from build123d import *

# Parameters (mm, degrees)
F0_R     = 4
F0_R_2   = 1.5
F1_DEPTH = 2
F2_DEPTH = 15
F3_SIZE  = 0.5
F4_W     = 2
F4_H     = 1
F5_DEPTH = 4.001
F6_DEPTH = 25.4


with BuildPart() as f1:
    # F0 (on Top) → F1 (new body)
    with BuildSketch(Plane.XY):
        Circle(F0_R)
        Circle(F0_R_2, mode=Mode.SUBTRACT)
    extrude(amount=F1_DEPTH)

    # F0 (on Top) → F2 (join)
    with BuildSketch(Plane.XY):
        Circle(F0_R_2)
    extrude(amount=F2_DEPTH)

    # F3
    f3_edges = [f1.edges().sort_by_distance(p)[0] for p in [
        (-4, 0, 2),
    ]]
    chamfer(f3_edges, length=F3_SIZE)

    # F4 (on Front) → F5 (cut, through all)
    with BuildSketch(Plane.XZ):
        with Locations((0.083052, 13.76275)):
            Rectangle(F4_W, F4_H)
    extrude(amount=-F5_DEPTH, mode=Mode.SUBTRACT)

    # F4 (on Front) → F6 (cut)
    with BuildSketch(Plane.XZ):
        with Locations((0.083052, 13.76275)):
            Rectangle(F4_W, F4_H)
    extrude(amount=F6_DEPTH, mode=Mode.SUBTRACT)


solid = f1.part
Input: part model. Units: mm. Frame: model coordinates. A direction names the side the tool comes from. Coordinates: 2 decimals unless noted, no trailing zeros. Order: outer loops, then holes, each group sorted by start corner. A loop starts at its lowest first (then second) coordinate and runs counter-clockwise, first axis right, second up. Notation, with made-up numbers: M 69.25,68 L 127.25,68 A18 ccw 127.25,88 Z; hole C 29.5,84 d3. An arc over 180 degrees is marked long. One line per question, with ' | ' between items.
Item 1: Pin query (flat end, axial travel): pin 1 (0.8 mm diameter, centred on y = 0, z = 13.5, fed in from +X); pin 2 (3 mm diameter, centred on x = -2.5, z = 9.5, fed in from +Y); pin 3 (4 mm diameter, centred on x = 0, z = 8.5, fed in from +Y). Return the tip coordinate at first contact, or that it passes through.
Geometry results:
pin 1: stops at x = 1.5 | pin 2: stops at y = 1.12 | pin 3: stops at y = 1.5
Item 2: Ray query, line 1 along Z through (x, y) = (-0.5, 0.5); line 2 along Z through (x, y) = (-0.75, 2.75); line 3 along X through (y, z) = (-1, 4.5). Return the intervals inside material, ascending.
Geometry results:
line 1: z = 0 to 13.26, 14.26 to 15 | line 2: z = 0 to 2 | line 3: x = -1.12 to 1.12
Item 3: Section A-A (x = 0). Output: boundary loops of the cut face in (y, z), then the cut area to 4 significant figures.
Geometry results:
outline: M -4,0 L 4,0 L 4,1.5 L 3.5,2 L 1.5,2 L 1.5,13.26 L -1.5,13.26 L -1.5,2 L -3.5,2 L -4,1.5 Z; M -1.5,14.26 L 1.5,14.26 L 1.5,15 L -1.5,15 Z | area: 51.75 mm^2
Item 4: Section C-C (z = 2.5). Output: boundary loops of the cut face in (x, y), then the cut area to 3 significant figures.
Geometry results:
outline: C 0,0 d3 | area: 7.07 mm^2
Item 5: Section B-B (y = 0). Output: boundary loops of the cut face in (x, z).
Geometry results:
outline: M -4,0 L 4,0 L 4,1.5 L 3.5,2 L 1.5,2 L 1.5,15 L -1.5,15 L -1.5,2 L -3.5,2 L -4,1.5 Z; hole M -0.92,13.26 L 1.08,13.26 L 1.08,14.26 L -0.92,14.26 Z
Item 6: Draft query along X for faces 4 (the flat face through (1.083, 0, 14)), 5 (the cylindrical face through (-0.867, -3.905, 0.74)), 6 (the flat face through (0, 0, 0)). Return one class per face: released by +X, released by -X, zero draft, split by the parting line, or undercut.
Geometry results:
face 4: undercut | face 5: split by the parting line | face 6: zero draft
Item 7: Reachability of faces 1 (the flat face through (0, 0, 15)), 2 (the cylindrical face through (-1.5, 0.07, 8.41)), 3 (the flat face through (0, 0, 14.263)) from +Z, -Z, +X, -X, +Y, -Y: full face, straight path, thin tool, end or side. Return the list, or none.
Geometry results:
face 1: +Z, +X, -X, +Y, -Y | face 2: +Z | face 3: +Y, -Y
